Work out the finished part from the listing and answer in its coordinate system (mm). A direction names the side the tool comes from. Give positions to 0.01 mm unless a question says otherwise; leave off trailing zeros. Write each loop counter-clockwise with the first axis right and the second up, starting at its lowest first coordinate (ties: lowest second). Pieces come first, ordered by that corner, then holes.
1) Find section A-A (z = 9.25). Determine the outline of the cut face in (x, y), plus the area to 3 significant figures.
2) Straight lines are drawn through the part: probe 1 along Y at (x, z) = (-206, 11.25); probe 2 along X at (y, z) = (-0.5, 7); probe 3 along X at (y, z) = (57, 8). For each, find the intervals that lie inside material, in ascending order.
3) A tool of negligible diameter and unlimited length cuts with its end or side. For faces 1 (the face through (-229, 101, 0)), 2 (the face through (-453.443, 122.43, 9.569)), from which of +Z, -Z, +X, -X, +Y, -Y can it reach the whole face along a straight path? Write none if from no direction.
4) Given pin 1 Ø1.9 at (y, z) = (45.5, 11) entering from -X; pin 2 Ø6 at (x, z) = (-409.5, 4.5) entering from +Y; pin 3 Ø3 at (x, z) = (-460, 8.5) entering from +Y, each flat-ended and moving along its own axis, determine where each tip first touches the part or whether it passes through.
5) Find section B-B (x = -27). Determine the outline of the cut face in (y, z).
6) Determine the mould class of faces 3 (the face through (-229, 101, 12.7)), 4 (the face through (-448.47, 118.17, 9.57)), 5 (the face through (-457.269, 125.708, 6.261)) for opening direction Y: pulls with the +Y half, pulls with the -Y half, needs draft (parallel to the pull), parting line crosses it, or undercut.
7) Find section C-C (y = 165). Determine the outline of the cut face in (x, z), plus the area to 3 significant figures.
```python
from build123d import *

# Parameters (mm, degrees)
BOSS_EXTRUDE1_DEPTH = 12.7
CUT_EXTRUDE1_DEPTH  = 6.35
SKETCH5_W           = 41.48623644
SKETCH5_H           = 6.5
CUT_EXTRUDE2_DEPTH  = 6.35


with BuildPart() as part:
    # Sketch1 → Boss-Extrude1 (new body)
    with BuildSketch(Plane.XY):
        Polygon((-524.529885057, -25.691954023), (75.470114943, -25.691954023), (75.470114943, 224.308045977), (-391.864893443, 224.308045977), (-524.529885057, 24.308045977), align=None)
    extrude(amount=BOSS_EXTRUDE1_DEPTH)

    # Sketch4 → Cut-Extrude1 (cut)
    with BuildSketch(Plane.XY.offset(12.7)):
        Polygon((-519.529885057, 22.800489254), (-519.529885057, -20.691954023), (70.470114943, -20.691954023), (70.470114943, 219.308045977), (-389.181518234, 219.308045977), align=None)
        Polygon((-513.029885057, 20.840665514), (-513.029885057, -14.191954023), (63.970114943, -14.191954023), (63.970114943, 212.808045977), (-385.693130461, 212.808045977), align=None, mode=Mode.SUBTRACT)
    extrude(amount=-CUT_EXTRUDE1_DEPTH, mode=Mode.SUBTRACT)

    # Sketch5 → Cut-Extrude2 (cut)
    with BuildSketch(Plane.XY.offset(12.7)):
        with Locations((65.370018612, 216.058045977)):
            Rectangle(SKETCH5_W, SKETCH5_H)
    extrude(amount=-CUT_EXTRUDE2_DEPTH, mode=Mode.SUBTRACT)


solid = part.part
```
Results:
1. outline: (-524.53, -25.69) - (75.47, -25.69) - (75.47, 212.81) - (70.47, 212.81) - (70.47, -20.69) - (-519.53, -20.69) - (-519.53, 22.8) - (-389.18, 219.31) - (75.47, 219.31) - (75.47, 224.31) - (-391.86, 224.31) - (-524.53, 24.31) - close; (-513.03, -14.19) - (63.97, -14.19) - (63.97, 212.81) - (-385.69, 212.81) - (-513.03, 20.84) - close
1. area: 127,000 mm2
2. probe 1: y = -25.69 to -20.69, -14.19 to 212.81, 219.31 to 224.31
2. probe 2: x = -524.53 to -519.53, -513.03 to 63.97, 70.47 to 75.47
2. probe 3: x = -502.84 to -496.84, -489.04 to 63.97, 70.47 to 75.47
3. face 1: -Z, +X, -X, +Y, -Y
3. face 2: +Z
4. pin 1: stops at x = -511.1
4. pin 2: stops at y = 202.24
4. pin 3: stops at y = 123.85
5. outline: (-25.69, 0) - (224.31, 0) - (224.31, 12.7) - (219.31, 12.7) - (219.31, 6.35) - (212.81, 6.35) - (212.81, 12.7) - (-14.19, 12.7) - (-14.19, 6.35) - (-20.69, 6.35) - (-20.69, 12.7) - (-25.69, 12.7) - close
6. face 3: needs draft
6. face 4: undercut
6. face 5: pulls with the +Y half
7. outline: (-431.21, 0) - (75.47, 0) - (75.47, 12.7) - (70.47, 12.7) - (70.47, 6.35) - (63.97, 6.35) - (63.97, 12.7) - (-417.41, 12.7) - (-417.41, 6.35) - (-425.21, 6.35) - (-425.21, 12.7) - (-431.21, 12.7) - close
7. area: 6,340 mm2
